from build123d import *

# Parameters (mm, degrees)
BOSS_EXTRUDE1_DEPTH             = 12.7
SHELL1_START                    = 2.54
SHELL1_DEPTH                    = 10.16
BOSS_EXTRUDE7_DEPTH             = 2.54
SKETCH7_W                       = 17.498012995
SKETCH7_H                       = 10.16
CUT_EXTRUDE5_DEPTH              = 48.524856948
SKETCH13_R                      = 4.572
BOSS_EXTRUDE3_DEPTH             = 2.54
CUT_EXTRUDE7_DEPTH              = 34.365857316
CUT_EXTRUDE7_DEPTH_BACK         = 34.365857316
SKETCH14_R                      = 2.667
F_8_32_TAPPED_HOLE1_D           = 3.4544
F_8_32_TAPPED_HOLE1_CSINK_D     = 5.4356
F_8_32_TAPPED_HOLE1_CSINK_ANGLE = 90
BOSS_EXTRUDE4_DEPTH             = 12.7
BOSS_EXTRUDE4_DEPTH_BACK        = 1.27
SKETCH18_R                      = 3.175
SKETCH19_R                      = 3.937
CUT_EXTRUDE8_DEPTH              = 2.54
FILLET1_R                       = 1.27


# Read off the part's stored shape, not the designer's step: Shell1
with BuildPart() as part:
    # Sketch1 → Boss-Extrude1 (new body)
    with BuildSketch(Plane.XY):
        with BuildLine():
            Line((17.500007037, 7.168559726), (15.574433037, 7.168559726))
            ThreePointArc((15.574433037, 7.168559726), (0, 19.486736174), (-15.574433037, 7.168559726))
            Line((-15.574433037, 7.168559726), (-17.500007037, 7.168559726))
            ThreePointArc((-17.500007037, 7.168559726), (-22.528950465, 5.085503154), (-24.612007037, 0.056559726))
            Line((-24.612007037, 0.056559726), (-24.612007037, -0.056559726))
            ThreePointArc((-24.612007037, -0.056559726), (-22.528950465, -5.085503154), (-17.500007037, -7.168559726))
            Line((-17.500007037, -7.168559726), (-15.574433037, -7.168559726))
            Line((-15.574433037, -7.168559726), (-10.470235042, -19.960271007))
            Line((-10.470235042, -19.960271007), (10.470222973, -19.960271007))
            Line((10.470222973, -19.960271007), (15.574433037, -7.168559726))
            Line((15.574433037, -7.168559726), (17.500007037, -7.168559726))
            ThreePointArc((17.500007037, -7.168559726), (22.548907748, -5.065466355), (24.611782132, 0))
            Line((24.611782132, 0), (24.611782132, 0.113119452))
            ThreePointArc((24.611782132, 0.113119452), (22.508913666, 5.105460437), (17.500007037, 7.168559726))
        make_face()
    extrude(amount=BOSS_EXTRUDE1_DEPTH)

    # Shell1 outline → Shell1 (cut)
    with BuildSketch(Plane.XY.offset(SHELL1_START)):
        with BuildLine():
            ThreePointArc((13.415909513, 4.628559726), (0, 16.946736174), (-13.415909513, 4.628559726))
            Line((-13.415909513, 4.628559726), (-17.500007037, 4.628559726))
            ThreePointArc((-17.500007037, 4.628559726), (-20.732899241, 3.28945193), (-22.072007037, 0.056559726))
            Line((-22.072007037, 0.056559726), (-22.072007037, -0.056559726))
            ThreePointArc((-22.072007037, -0.056559726), (-20.732899241, -3.28945193), (-17.500007037, -4.628559726))
            Line((-17.500007037, -4.628559726), (-13.853209773, -4.628559726))
            Line((-13.853209773, -4.628559726), (-8.749011778, -17.420271007))
            Line((-8.749011778, -17.420271007), (8.749001217, -17.420271007))
            Line((8.749001217, -17.420271007), (13.853211281, -4.628559726))
            Line((13.853211281, -4.628559726), (17.500007037, -4.628559726))
            ThreePointArc((17.500007037, -4.628559726), (20.748892784, -3.273378869), (22.071782132, -0.011211257))
            Line((22.071782132, -0.011211257), (22.071782132, 0.101908195))
            ThreePointArc((22.071782132, 0.101908195), (20.71682618, 3.305445473), (17.500007037, 4.628559726))
            Line((17.500007037, 4.628559726), (13.415909513, 4.628559726))
        make_face()
    extrude(amount=SHELL1_DEPTH, mode=Mode.SUBTRACT)

    # Sketch22 → Boss-Extrude7 (add)
    with BuildSketch(Plane(origin=(0, 0, 0), x_dir=(-1, 0, 0), z_dir=(0, 0, -1))):
        with BuildLine():
            Line((-17.28751812, 7.168559726), (17.136892248, 7.168559726))
            ThreePointArc((17.136892248, 7.168559726), (-0.075312936, 21.200593012), (-17.28751812, 7.168559726))
        make_face()
    extrude(amount=-BOSS_EXTRUDE7_DEPTH)

    # Sketch7 → Cut-Extrude5 (cut, through all)
    with BuildSketch(Plane(origin=(0, -17.420271007, 0), x_dir=(1, 0, 0), z_dir=(0, 1, 0))):
        with Locations((-5.28e-06, -7.62)):
            Rectangle(SKETCH7_W, SKETCH7_H)
    extrude(amount=-CUT_EXTRUDE5_DEPTH, mode=Mode.SUBTRACT)

    # Sketch13 → Boss-Extrude3 (add)
    with BuildSketch(Plane.XY.offset(2.54)):
        with BuildLine():
            Line((-17.500007037, -4.628559726), (-13.852164447, -4.628559726))
            ThreePointArc((-13.852164447, -4.628559726), (0, -14.605), (13.852164447, -4.628559726))
            Line((13.852164447, -4.628559726), (16.51, -4.628559726))
            ThreePointArc((16.51, -4.628559726), (21.991424378, -1.364408419), (19.119271672, 4.332207752))
            ThreePointArc((19.119271672, 4.332207752), (18.323086992, 4.553861516), (17.500007037, 4.628559726))
            Line((17.500007037, 4.628559726), (13.415909513, 4.628559726))
            ThreePointArc((13.415909513, 4.628559726), (0, 16.946736174), (-13.415909513, 4.628559726))
            Line((-13.415909513, 4.628559726), (-16.51, 4.628559726))
            ThreePointArc((-16.51, 4.628559726), (-21.991424378, 1.364408419), (-19.119271672, -4.332207752))
            ThreePointArc((-19.119271672, -4.332207752), (-18.323086992, -4.553861516), (-17.500007037, -4.628559726))
        make_face()
        with Locations((0, 8.509)):
            Circle(SKETCH13_R, mode=Mode.SUBTRACT)
    extrude(amount=BOSS_EXTRUDE3_DEPTH)

    # Sketch14 → Cut-Extrude7 (cut, two sides: drawn at the far end of the back side and taken through both)
    with BuildSketch(Plane.XY.offset(5.08).offset(-CUT_EXTRUDE7_DEPTH_BACK)):
        with Locations((0, 8.50001094)):
            Circle(SKETCH14_R)
    extrude(amount=CUT_EXTRUDE7_DEPTH + CUT_EXTRUDE7_DEPTH_BACK, mode=Mode.SUBTRACT)

    # #8-32 Tapped Hole1 (through all)
    with Locations(Plane.XY.offset(5.08)):
        with Locations((-17.500007037, 0), (17.500007037, 0)):
            CounterSinkHole(F_8_32_TAPPED_HOLE1_D / 2, F_8_32_TAPPED_HOLE1_CSINK_D / 2, counter_sink_angle=F_8_32_TAPPED_HOLE1_CSINK_ANGLE)

    # Sketch18 → Boss-Extrude4 (add, two sides: drawn at the far end of the back side and taken through both)
    with BuildSketch(Plane(origin=(0, 19.486736174, 0), x_dir=(1, 0, 0), z_dir=(0, 1, 0)).offset(-BOSS_EXTRUDE4_DEPTH_BACK)):
        with Locations(Location((0, -8.89, 0), (0, 0, 270))):
            Circle(SKETCH18_R)
    extrude(amount=BOSS_EXTRUDE4_DEPTH + BOSS_EXTRUDE4_DEPTH_BACK)

    # Sketch19 → Cut-Extrude8 (cut)
    with BuildSketch(Plane(origin=(0, 0, 0), x_dir=(-1, 0, 0), z_dir=(0, 0, -1))):
        with Locations((0, 8.50001094)):
            Circle(SKETCH19_R)
    extrude(amount=-CUT_EXTRUDE8_DEPTH, mode=Mode.SUBTRACT)

    # Fillet1
    fillet1_edges = [part.edges().sort_by_distance(p)[0] for p in [
        (13.415909513, 4.628559726, 8.89),
        (-13.415909513, 4.628559726, 8.89),
    ]]
    fillet(fillet1_edges, radius=FILLET1_R)


solid = part.part
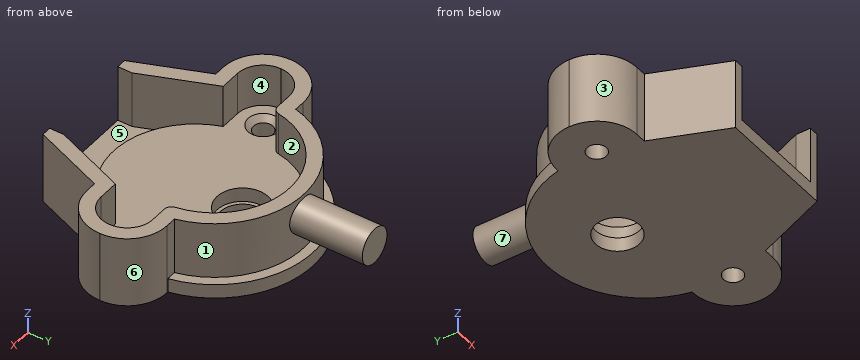
Design review of the part built by this model. Coordinates are the model's own, in mm. Face numbers are marked on the shaded views. A direction names the side the tool comes from. Coordinates: 2 decimals unless noted, no trailing zeros. Write each loop counter-clockwise with the first axis right and the second up, starting at its lowest first coordinate (ties: lowest second). Pieces come first, ordered by that corner, then holes. Notation, with made-up numbers: (67.25, -19) - (98.25, -19) arc R26 ccw to (98.25, 11) - close; hole circle Ø5 at (55.5, 23). An arc over 180 degrees is marked (long way). One line per item, written item: value.
1) For the marked faces 5, 6 and 7, list the 3-axis set-ups (+Z, -Z, +X, -X, +Y, -Y) from which the entire face can be reached by the end or side of a thin tool; tool diameter is ignored.
Answer sheet:
face 5: +Z
face 6: +Z, -Z, +X, +Y
face 7: +Y
2) Add section D-D (x = 6). State the section outline as (y, z) points.
Answer sheet:
outline: (-19.96, 0) - (20.17, 0) - (20.17, 2.54) - (18.32, 2.54) - (18.32, 12.7) - (15.54, 12.7) - (15.54, 5.08) - (-13.32, 5.08) - (-13.32, 2.54) - (-19.96, 2.54) - close
3) Mouldability with a two-part tool opening along X and no side actions: class the marked faces 1, 2, 3 and 4 as +X half, -X half, draft (parallel to the pull), parting line (faces both ways), or undercut.
Answer sheet:
face 1: parting line
face 2: undercut
face 3: -X half
face 4: undercut
4) Add section B-B (x = 11.5). State the section outline as (y, z) points, plus the area to 3 significant figures.
Answer sheet:
outline: (-17.38, 0) - (16.98, 0) - (16.98, 2.54) - (14.61, 2.54) - (14.61, 12.7) - (10.49, 12.7) - (10.49, 5.08) - (-9, 5.08) - (-9, 2.54) - (-10.53, 2.54) - (-10.53, 12.7) - (-17.38, 12.7) - close
area: 248 mm2
5) Add section A-A (y = -13). State the section outline as (x, z) points, plus the area to 3 significant figures.
Answer sheet:
outline: (-13.25, 0) - (13.25, 0) - (13.25, 12.7) - (10.51, 12.7) - (10.51, 2.54) - (6.66, 2.54) - (6.66, 5.08) - (-6.66, 5.08) - (-6.66, 2.54) - (-10.51, 2.54) - (-10.51, 12.7) - (-13.25, 12.7) - close
area: 157 mm2
6) Insertion check: pin 1 (4 mm diameter, centred on x = 15, z = 9, fed in from +Y); pin 2 (4 mm diameter, centred on y = -5, z = 2, fed in from +X); pin 3 (0.8 mm diameter, centred on y = -19, z = 8, fed in from -X). Each pin has a flat end and moves straight along its axis. Give the tip position at first contact, or say it passes through.
Answer sheet:
pin 1: stops at y = 12.82
pin 2: stops at x = 23.97
pin 3: stops at x = -11.01
7) To check wall thickness, follow probe 1 along Z at (x, y) = (-7, 12.5); probe 2 along X at (y, z) = (1, 8); probe 3 along Y at (x, z) = (0, 2.5). State the ranges of each line that lie inside material, in increasing order.
Answer sheet:
probe 1: z = 0 to 5.08
probe 2: x = -24.55 to -21.97, 21.97 to 24.55
probe 3: y = -19.96 to 4.56, 12.44 to 21.2
